The listing builds one solid part. Answer for the finished solid, in the listing's coordinates (mm). Face numbers are marked on the shaded views. A direction names the side the tool comes from. Coordinates: 2 decimals unless noted, no trailing zeros. Write each loop counter-clockwise with the first axis right and the second up, starting at its lowest first coordinate (ties: lowest second). Pieces come first, ordered by that corner, then holes.
(1) The part is cut by section A-A on y = -24.5. Determine the outline of the cut face in (x, z).
(2) The part is cut by section B-B on z = 8.25. Determine the outline of the cut face in (x, y).
(3) For a pull along X with two mould halves and no side action, classify the marked faces 1, 2 and 3 as +X half, -X half, draft (parallel to the pull), parting line (faces both ways), or undercut.
(4) The part is cut by section C-C on z = 14.25. Determine the outline of the cut face in (x, y).
(5) Which of the six approach directions +Z, -Z, +X, -X, +Y, -Y give full straight-line access (tool end or side, diameter ignored) to the marked faces 4, 5, 6, 7 and 8?
(6) Given P1, Ø5, axis at x = 33, y = -40, coming from the +Z side; P2, Ø8, axis at x = -23.5, y = -6.5, coming from the -Z side; P3, Ø8, axis at y = -6.5, z = 10, coming from the +X side, each flat-ended and moving along its own axis, determine where each tip first touches the part or whether it passes through.
(7) The part is cut by section D-D on x = 24.4. Determine the outline of the cut face in (y, z), plus the area to 3 significant figures.
(8) Straight lines are drawn through the part: line 1 (X direction, y = -24.6, z = 8.25); line 2 (Y direction, x = 31.75, z = -2.05); line 3 (X direction, y = -14.5, z = 9.5). For each, find the intervals that lie inside material, in ascending order.
from build123d import *

# Parameters (mm, degrees)
EXTRUDE_1_DEPTH     = 16.5
SKETCH_2_R          = 2.5
CUT_EXTRUDE_1_DEPTH = 16.5
SKETCH_3_W          = 10
SKETCH_3_H          = 16.5
CUT_EXTRUDE_2_DEPTH = 3
SKETCH_5_R          = 2
CUT_EXTRUDE_4_DEPTH = 48.945933091
SKETCH_6_W          = 10
SKETCH_6_H          = 23
EXTRUDE_2_DEPTH     = 3
SKETCH_7_R          = 2.5
CUT_EXTRUDE_5_DEPTH = 3
SKETCH2_W           = 16.5
SKETCH2_H           = 23
BOSS_EXTRUDE1_DEPTH = 1
SKETCH3_W           = 16.5
SKETCH3_H           = 23
BOSS_EXTRUDE2_DEPTH = 1


with BuildPart() as part:
    # 草图1 → 凸台-拉伸1 (new body)
    with BuildSketch(Plane.XY):
        Polygon((0, 0), (26.75, 0), (26.75, -20), (36.75, -20), (36.75, -26), (20.75, -26), (20.75, -6), (0, -6), (-20.75, -6), (-20.75, -26), (-36.75, -26), (-36.75, -20), (-26.75, -20), (-26.75, 0), align=None)
    extrude(amount=EXTRUDE_1_DEPTH)

    # 草图2 → 切除-拉伸1 (cut)
    with BuildSketch(Plane(origin=(0, -20, 0), x_dir=(1, 0, 0), z_dir=(0, 1, 0))):
        with Locations(Location((32.75, -8.25, 0), (0, 0, 270))):
            Circle(SKETCH_2_R)
        with Locations(Location((-32.75, -8.25, 0), (0, 0, 270))):
            Circle(SKETCH_2_R)
    extrude(amount=-CUT_EXTRUDE_1_DEPTH, mode=Mode.SUBTRACT)

    # 草图3 → 切除-拉伸2 (cut)
    with BuildSketch(Plane(origin=(0, -20, 0), x_dir=(1, 0, 0), z_dir=(0, 1, 0))):
        with Locations((31.75, -8.25)):
            Rectangle(SKETCH_3_W, SKETCH_3_H)
        with Locations((-31.75, -8.25)):
            Rectangle(SKETCH_3_W, SKETCH_3_H)
    extrude(amount=-CUT_EXTRUDE_2_DEPTH, mode=Mode.SUBTRACT)

    # 草图5 → 切除-拉伸4 (cut, through all)
    with BuildSketch(Plane(origin=(0, 0, 0), x_dir=(-1, 0, 0), z_dir=(0, 0, -1))):
        with Locations((-24.4, -11)):
            Circle(SKETCH_5_R)
        with Locations((-24.4, -21)):
            Circle(SKETCH_5_R)
        with Locations(Location((24.4, -21, 0), (0, 0, 180))):
            Circle(SKETCH_5_R)
        with Locations(Location((24.4, -11, 0), (0, 0, 180))):
            Circle(SKETCH_5_R)
    extrude(amount=-CUT_EXTRUDE_4_DEPTH, mode=Mode.SUBTRACT)

    # 草图6 → 凸台-拉伸2 (add)
    with BuildSketch(Plane(origin=(0, 0, 0), x_dir=(-1, 0, 0), z_dir=(0, 0, -1))):
        with Locations((-31.75, -34.5)):
            Rectangle(SKETCH_6_W, SKETCH_6_H)
        with Locations((31.75, -34.5)):
            Rectangle(SKETCH_6_W, SKETCH_6_H)
    extrude(amount=EXTRUDE_2_DEPTH)

    # 草图7 → 切除-拉伸5 (cut)
    with BuildSketch(Plane(origin=(0, 0, -3), x_dir=(-1, 0, 0), z_dir=(0, 0, -1))):
        with Locations((-31.75, -36)):
            Circle(SKETCH_7_R)
        with Locations((31.75, -36)):
            Circle(SKETCH_7_R)
    extrude(amount=-CUT_EXTRUDE_5_DEPTH, mode=Mode.SUBTRACT)

    # Sketch2 → Boss-Extrude1 (add)
    with BuildSketch(Plane.ZY.offset(26.75)):
        with Locations((8.25, -11.5)):
            Rectangle(SKETCH2_W, SKETCH2_H)
    extrude(amount=BOSS_EXTRUDE1_DEPTH)

    # Sketch3 → Boss-Extrude2 (add)
    with BuildSketch(Plane(origin=(26.75, 0, 0), x_dir=(0, 0, -1), z_dir=(1, 0, 0))):
        with Locations((-8.25, -11.5)):
            Rectangle(SKETCH3_W, SKETCH3_H)
    extrude(amount=BOSS_EXTRUDE2_DEPTH)


solid = part.part
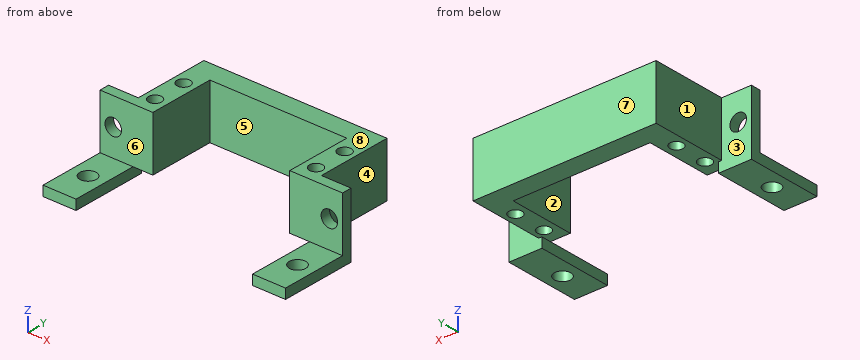
Model answer:
1. outline: (-36.75, -3) - (-26.75, -3) - (-26.75, 0) - (-20.75, 0) - (-20.75, 16.5) - (-36.75, 16.5) - close; (20.75, 0) - (26.75, 0) - (26.75, -3) - (36.75, -3) - (36.75, 16.5) - (20.75, 16.5) - close; hole circle Ø5 at (-32.75, 8.25); hole circle Ø5 at (32.75, 8.25)
2. outline: (-36.75, -26) - (-35.25, -26) - (-35.25, -23) - (-36.75, -23) - close; (-30.25, -26) - (-20.75, -26) - (-20.75, -6) - (20.75, -6) - (20.75, -26) - (30.25, -26) - (30.25, -23) - (27.75, -23) - (27.75, 0) - (-27.75, 0) - (-27.75, -23) - (-30.25, -23) - close; (35.25, -26) - (36.75, -26) - (36.75, -23) - (35.25, -23) - close; hole circle Ø4 at (-24.4, -21); hole circle Ø4 at (-24.4, -11); hole circle Ø4 at (24.4, -21); hole circle Ø4 at (24.4, -11)
3. face 1: -X half
3. face 2: undercut
3. face 3: draft
4. outline: (-36.75, -26) - (-20.75, -26) - (-20.75, -6) - (20.75, -6) - (20.75, -26) - (36.75, -26) - (36.75, -23) - (27.75, -23) - (27.75, 0) - (-27.75, 0) - (-27.75, -23) - (-36.75, -23) - close; hole circle Ø4 at (-24.4, -21); hole circle Ø4 at (-24.4, -11); hole circle Ø4 at (24.4, -21); hole circle Ø4 at (24.4, -11)
5. face 4: +Z, -Z, +X, +Y
5. face 5: +Z, -Z, -Y
5. face 6: +Z, +X, -X, -Y
5. face 7: +Z, -Z, +X, -X, +Y
5. face 8: +Z, +X, -X, +Y, -Y
6. P1: stops at z = 0
6. P2: stops at z = 0
6. P3: stops at x = 27.75
7. outline: (-26, 0) - (-23, 0) - (-23, 16.5) - (-26, 16.5) - close; (-19, 0) - (-13, 0) - (-13, 16.5) - (-19, 16.5) - close; (-9, 0) - (0, 0) - (0, 16.5) - (-9, 16.5) - close
7. area: 297 mm2
8. line 1: x = -36.75 to -35.25, -30.25 to -20.75, 20.75 to 30.25, 35.25 to 36.75
8. line 2: y = -46 to -38.5, -33.5 to -23
8. line 3: x = -27.75 to -20.75, 20.75 to 27.75
